```python
from build123d import *

# Parameters (mm, degrees)
BOSS_EXTRUDE1_DEPTH = 10
CUT_EXTRUDE1_REACH  = 172.294
SKETCH2_R           = 2.5


with BuildPart() as part:
    # Sketch1 → Boss-Extrude1 (new body)
    with BuildSketch(Plane.XY):
        Polygon((0, 0), (40, 0), (80, 40), (80, 80), (40, 150), (0, 150), align=None)
    extrude(amount=BOSS_EXTRUDE1_DEPTH)

    # Sketch2 → Cut-Extrude1 (cut, up to next)
    with BuildSketch(Plane.XY.offset(10), mode=Mode.PRIVATE) as cut_extrude1_sk1:
        with Locations((10, 10)):
            Circle(SKETCH2_R)
    cut_extrude1_tool1 = extrude(cut_extrude1_sk1.sketch, amount=-CUT_EXTRUDE1_REACH, mode=Mode.PRIVATE) & part.part
    # Sketch2 → Cut-Extrude1 (cut, up to next)
    with BuildSketch(Plane.XY.offset(10), mode=Mode.PRIVATE) as cut_extrude1_sk2:
        with Locations((30, 10)):
            Circle(SKETCH2_R)
    cut_extrude1_tool2 = extrude(cut_extrude1_sk2.sketch, amount=-CUT_EXTRUDE1_REACH, mode=Mode.PRIVATE) & part.part
    # Sketch2 → Cut-Extrude1 (cut, up to next)
    with BuildSketch(Plane.XY.offset(10), mode=Mode.PRIVATE) as cut_extrude1_sk3:
        with Locations((10, 50)):
            Circle(SKETCH2_R)
    cut_extrude1_tool3 = extrude(cut_extrude1_sk3.sketch, amount=-CUT_EXTRUDE1_REACH, mode=Mode.PRIVATE) & part.part
    # Sketch2 → Cut-Extrude1 (cut, up to next)
    with BuildSketch(Plane.XY.offset(10), mode=Mode.PRIVATE) as cut_extrude1_sk4:
        with Locations((70, 70)):
            Circle(SKETCH2_R)
    cut_extrude1_tool4 = extrude(cut_extrude1_sk4.sketch, amount=-CUT_EXTRUDE1_REACH, mode=Mode.PRIVATE) & part.part
    # Sketch2 → Cut-Extrude1 (cut, up to next)
    with BuildSketch(Plane.XY.offset(10), mode=Mode.PRIVATE) as cut_extrude1_sk5:
        with Locations((50, 70)):
            Circle(SKETCH2_R)
    cut_extrude1_tool5 = extrude(cut_extrude1_sk5.sketch, amount=-CUT_EXTRUDE1_REACH, mode=Mode.PRIVATE) & part.part
    # Sketch2 → Cut-Extrude1 (cut, up to next)
    with BuildSketch(Plane.XY.offset(10), mode=Mode.PRIVATE) as cut_extrude1_sk6:
        with Locations((50, 50)):
            Circle(SKETCH2_R)
    cut_extrude1_tool6 = extrude(cut_extrude1_sk6.sketch, amount=-CUT_EXTRUDE1_REACH, mode=Mode.PRIVATE) & part.part
    # Sketch2 → Cut-Extrude1 (cut, up to next)
    with BuildSketch(Plane.XY.offset(10), mode=Mode.PRIVATE) as cut_extrude1_sk7:
        with Locations((30, 50)):
            Circle(SKETCH2_R)
    cut_extrude1_tool7 = extrude(cut_extrude1_sk7.sketch, amount=-CUT_EXTRUDE1_REACH, mode=Mode.PRIVATE) & part.part
    # Sketch2 → Cut-Extrude1 (cut, up to next)
    with BuildSketch(Plane.XY.offset(10), mode=Mode.PRIVATE) as cut_extrude1_sk8:
        with Locations((70, 50)):
            Circle(SKETCH2_R)
    cut_extrude1_tool8 = extrude(cut_extrude1_sk8.sketch, amount=-CUT_EXTRUDE1_REACH, mode=Mode.PRIVATE) & part.part
    # Sketch2 → Cut-Extrude1 (cut, up to next)
    with BuildSketch(Plane.XY.offset(10), mode=Mode.PRIVATE) as cut_extrude1_sk9:
        with Locations((30, 90)):
            Circle(SKETCH2_R)
    cut_extrude1_tool9 = extrude(cut_extrude1_sk9.sketch, amount=-CUT_EXTRUDE1_REACH, mode=Mode.PRIVATE) & part.part
    # Sketch2 → Cut-Extrude1 (cut, up to next)
    with BuildSketch(Plane.XY.offset(10), mode=Mode.PRIVATE) as cut_extrude1_sk10:
        with Locations((10, 90)):
            Circle(SKETCH2_R)
    cut_extrude1_tool10 = extrude(cut_extrude1_sk10.sketch, amount=-CUT_EXTRUDE1_REACH, mode=Mode.PRIVATE) & part.part
    # Sketch2 → Cut-Extrude1 (cut, up to next)
    with BuildSketch(Plane.XY.offset(10), mode=Mode.PRIVATE) as cut_extrude1_sk11:
        with Locations((10, 70)):
            Circle(SKETCH2_R)
    cut_extrude1_tool11 = extrude(cut_extrude1_sk11.sketch, amount=-CUT_EXTRUDE1_REACH, mode=Mode.PRIVATE) & part.part
    # Sketch2 → Cut-Extrude1 (cut, up to next)
    with BuildSketch(Plane.XY.offset(10), mode=Mode.PRIVATE) as cut_extrude1_sk12:
        with Locations((30, 70)):
            Circle(SKETCH2_R)
    cut_extrude1_tool12 = extrude(cut_extrude1_sk12.sketch, amount=-CUT_EXTRUDE1_REACH, mode=Mode.PRIVATE) & part.part
    add(cut_extrude1_tool1.solids().sort_by_distance((10, 10, 10))[0], mode=Mode.SUBTRACT)
    add(cut_extrude1_tool2.solids().sort_by_distance((30, 10, 10))[0], mode=Mode.SUBTRACT)
    add(cut_extrude1_tool3.solids().sort_by_distance((10, 50, 10))[0], mode=Mode.SUBTRACT)
    add(cut_extrude1_tool4.solids().sort_by_distance((70, 70, 10))[0], mode=Mode.SUBTRACT)
    add(cut_extrude1_tool5.solids().sort_by_distance((50, 70, 10))[0], mode=Mode.SUBTRACT)
    add(cut_extrude1_tool6.solids().sort_by_distance((50, 50, 10))[0], mode=Mode.SUBTRACT)
    add(cut_extrude1_tool7.solids().sort_by_distance((30, 50, 10))[0], mode=Mode.SUBTRACT)
    add(cut_extrude1_tool8.solids().sort_by_distance((70, 50, 10))[0], mode=Mode.SUBTRACT)
    add(cut_extrude1_tool9.solids().sort_by_distance((30, 90, 10))[0], mode=Mode.SUBTRACT)
    add(cut_extrude1_tool10.solids().sort_by_distance((10, 90, 10))[0], mode=Mode.SUBTRACT)
    add(cut_extrude1_tool11.solids().sort_by_distance((10, 70, 10))[0], mode=Mode.SUBTRACT)
    add(cut_extrude1_tool12.solids().sort_by_distance((30, 70, 10))[0], mode=Mode.SUBTRACT)


solid = part.part
```
The listing builds one solid part. Answer for the finished solid, in the listing's coordinates (mm). Give positions to 0.01 mm unless a question says otherwise; leave off trailing zeros. Write each loop counter-clockwise with the first axis right and the second up, starting at its lowest first coordinate (ties: lowest second). Pieces come first, ordered by that corner, then holes. Notation, with made-up numbers: M 82,7.25 L 130,7.25 A11 cw 130,28.25 Z; hole C -19,-39 d11. An arc over 180 degrees is marked long. Write each question's results on one line, items separated by ' | '.
Q1. Flat-ended cylindrical pins translate along their axes: P1, Ø4.5, axis at x = 50, y = 50, coming from the +Z side; P2, Ø4, axis at x = 64.5, z = 4.5, coming from the -Y side. Find the tip coordinate at first contact, or state that the pin passes through.
Output values:
P1: through | P2: y = 22.5
Q2. For a pull along Y with two mould halves and no side action, classify faces 1 (the flat face through (20, 150, 5)), 2 (the cylindrical face through (29.46, 67.56, 5.07)), 3 (the cylindrical face through (52.31, 69.04, 5.07)), 4 (the flat face through (31, 76, 0)) as released by +Y, released by -Y, zero draft, split by the parting line, or undercut.
Output values:
face 1: released by +Y | face 2: undercut | face 3: undercut | face 4: zero draft
Q3. Section B-B, the plane y = 70 is taken. Write down the section's boundary in (x, z).
Output values:
outline: M 0,0 L 7.5,0 L 7.5,10 L 0,10 Z; M 12.5,0 L 27.5,0 L 27.5,10 L 12.5,10 Z; M 32.5,0 L 47.5,0 L 47.5,10 L 32.5,10 Z; M 52.5,0 L 67.5,0 L 67.5,10 L 52.5,10 Z; M 72.5,0 L 80,0 L 80,10 L 72.5,10 Z
Q4. Section C-C, the plane x = 10 is taken. Write down the section's boundary in (y, z).
Output values:
outline: M 0,0 L 7.5,0 L 7.5,10 L 0,10 Z; M 12.5,0 L 47.5,0 L 47.5,10 L 12.5,10 Z; M 52.5,0 L 67.5,0 L 67.5,10 L 52.5,10 Z; M 72.5,0 L 87.5,0 L 87.5,10 L 72.5,10 Z; M 92.5,0 L 150,0 L 150,10 L 92.5,10 Z
Q5. Section D-D, the plane z = 5.5 is taken. Count the separate pieces of the cut face and the enclosed holes in it, then the cut area to 3 significant figures.
Output values:
separate pieces: 1 | enclosed holes: 12 | area: 9,560 mm2
Q6. Section A-A, the plane x = 50 is taken. Write down the section's boundary in (y, z), then the cut area to 4 significant figures.
Output values:
outline: M 10,0 L 47.5,0 L 47.5,10 L 10,10 Z; M 52.5,0 L 67.5,0 L 67.5,10 L 52.5,10 Z; M 72.5,0 L 132.5,0 L 132.5,10 L 72.5,10 Z | area: 1,125 mm2
Q7. Consider L1, parallel to Y at x = 30, z = 5.5; L2, parallel to Y at x = 68, z = 5.25; L3, parallel to Y at x = 50, z = 7. Determine where each line is inside the solid, lowest interval first. Write a range as from..to.
Output values:
L1: 0..7.5, 12.5..47.5, 52.5..67.5, 72.5..87.5, 92.5..150 | L2: 28..48.5, 51.5..68.5, 71.5..101 | L3: 10..47.5, 52.5..67.5, 72.5..132.5
